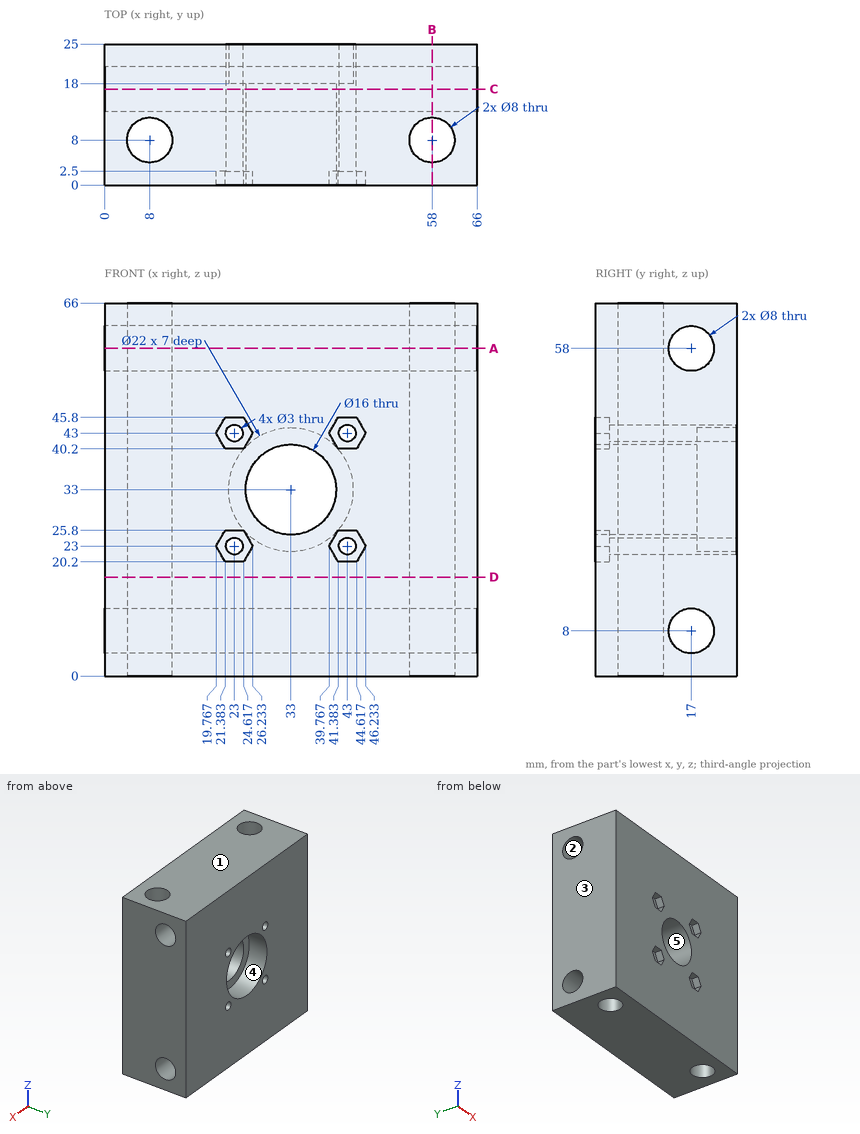
Source: three-view drawing plus pictorial views. Frame: mm from the lowest corner of the part. A direction names the side the tool comes from. Give positions to 0.01 mm unless a question says otherwise; leave off trailing zeros. Loops run counter-clockwise (first coordinate to the right, second up) from the corner with the lowest first, then second, coordinate; pieces in that order, holes last. Notation, with made-up numbers: M 71,11 L 128,11 A13 cw 128,20 Z; hole C 51,26.5 d11. An arc over 180 degrees is marked long. Put each result on its own line as item: value.
Q1. Reachability of the marked faces 4 and 5 from +Z, -Z, +X, -X, +Y, -Y: full face, straight path, thin tool, end or side. Return the list, or none.
Response values:
face 4: +Y
face 5: +Y, -Y
Q2. Section B-B (x = 58). Return the cut outline in (y, z), and give its area (3 significant figures).
Response values:
outline: M 0,0 L 4,0 L 4,66 L 0,66 Z; M 12,0 L 25,0 L 25,66 L 12,66 Z; hole C 17,8 d8; hole C 17,58 d8
area: 1,020 mm²
Q3. Line query: probe 1 along X at (y, z) = (15, 43); probe 2 along Y at (x, z) = (29, 8); probe 3 along X at (y, z) = (9.25, 28) (1 decimal). Output: solid intervals per line, ascending. Write a range as [from, to].
Response values:
probe 1: x = [0, 21.5], [24.5, 41.5], [44.5, 66]
probe 2: y = [0, 13], [21, 25]
probe 3: x = [0, 4.2], [11.8, 26.8], [39.2, 54.2], [61.8, 66]
Q4. Section D-D (z = 17.5). Return the cut outline in (x, y), and give its area (3 significant figures).
Response values:
outline: M 0,0 L 66,0 L 66,25 L 0,25 Z; hole C 8,8 d8; hole C 58,8 d8
area: 1,550 mm²
Q5. Section C-C (y = 17). Return the cut outline in (x, z), and give its area (3 significant figures).
Response values:
outline: M 0,0 L 66,0 L 66,4 L 0,4 Z; M 0,12 L 66,12 L 66,54 L 0,54 Z; M 0,62 L 66,62 L 66,66 L 0,66 Z; hole C 23,23 d3; hole C 23,43 d3; hole C 33,33 d16; hole C 43,23 d3; hole C 43,43 d3
area: 3,070 mm²
Q6. Pin query (flat end, axial travel): P1, Ø7, axis at x = 8, y = 8, coming from the -Z side; P2, Ø3, axis at x = 23, z = 24, coming from the -Y side. Return the tip coordinate at first contact, or that it passes through.
Response values:
P1: passes through
P2: stops at y = 2.5
Q7. Section A-A (z = 58). Return the cut outline in (x, y), and give its area (3 significant figures).
Response values:
outline: M 0,0 L 66,0 L 66,13 L 0,13 Z; M 0,21 L 66,21 L 66,25 L 0,25 Z; hole C 8,8 d8; hole C 58,8 d8
area: 1,020 mm²
Q8. Mould query, pull axis Z, two halves, no side actions, for the marked faces 1, 2 and 3. Classes: released by +Z, released by -Z, zero draft, split by the parting line, or undercut.
Response values:
face 1: released by +Z
face 2: undercut
face 3: zero draft
